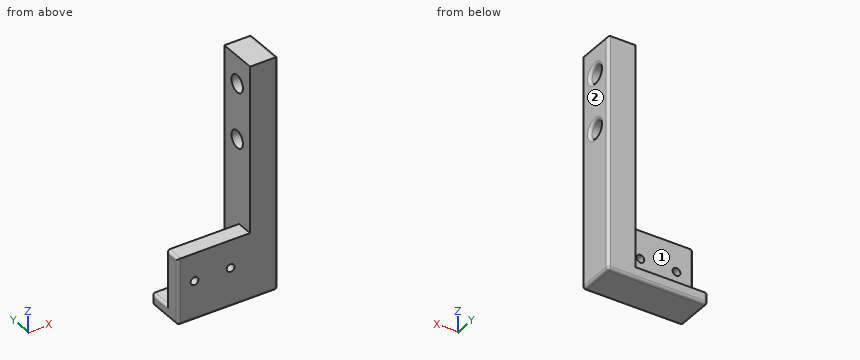
```python
from build123d import *

# Parameters (mm, degrees)
SKETCH_1_R          = 0.7
EXTRUDE_1_DEPTH     = 7
SKETCH_2_R          = 1.55
CUT_EXTRUDE_1_DEPTH = 32.591137998
SKETCH_3_W          = 13
SKETCH_3_H          = 10
CUT_EXTRUDE_2_DEPTH = 4
SKETCH_4_W          = 18
SKETCH_4_H          = 2
EXTRUDE_2_DEPTH     = 7
FILLET_1_R          = 0.5
FILLET_2_R          = 0.5


with BuildPart() as part:
    # 草图1 → 凸台-拉伸1 (new body)
    with BuildSketch(Plane(origin=(0, 0, 0), x_dir=(1, 0, 0), z_dir=(0, 1, 0))):
        Polygon((-2.5, 15), (-2.5, -15), (2.5, -15), (2.5, 15), (2.5, 25), (-15.5, 25), (-15.5, 15), align=None)
        with Locations(Location((-12.5, 20, 0), (0, 0, 270))):
            Circle(SKETCH_1_R, mode=Mode.SUBTRACT)
        with Locations(Location((-6, 20, 0), (0, 0, 270))):
            Circle(SKETCH_1_R, mode=Mode.SUBTRACT)
    extrude(amount=EXTRUDE_1_DEPTH)

    # 草图2 → 切除-拉伸1 (cut, through all)
    with BuildSketch(Plane(origin=(2.5, 0, 0), x_dir=(0, 0, -1), z_dir=(1, 0, 0))):
        with Locations((-10, 3.5)):
            Circle(SKETCH_2_R)
        with Locations((0, 3.5)):
            Circle(SKETCH_2_R)
    extrude(amount=-CUT_EXTRUDE_1_DEPTH, mode=Mode.SUBTRACT)

    # 草图3 → 切除-拉伸2 (cut)
    with BuildSketch(Plane(origin=(0, 7, 0), x_dir=(1, 0, 0), z_dir=(0, 1, 0))):
        with Locations((-9, 20)):
            Rectangle(SKETCH_3_W, SKETCH_3_H)
    extrude(amount=-CUT_EXTRUDE_2_DEPTH, mode=Mode.SUBTRACT)

    # 草图4 → 凸台-拉伸2 (add)
    with BuildSketch(Plane.XZ):
        with Locations((-6.5, -26)):
            Rectangle(SKETCH_4_W, SKETCH_4_H)
    extrude(amount=-EXTRUDE_2_DEPTH)

    # 圆角1
    fillet_1_edges = [part.edges().sort_by_distance(p)[0] for p in [
        (2.5, 3.5, 15),
        (2.5, 3.5, 11.55),
        (2.5, 3.5, 1.55),
        (2.5, 7, -6),
        (-15.5, 3.5, -27),
        (-6.5, 7, -27),
        (2.5, 3.5, -27),
        (-6.5, 0, -27),
        (2.5, 0, -6),
    ]]
    fillet(fillet_1_edges, radius=FILLET_1_R)

    # 圆角2
    # the kernel refuses this fillet: 0.5 mm, written as the material it takes off along each edge
    with BuildSketch(Plane(origin=(-15, 6.5, -26.5), x_dir=(-1, 0, 0), z_dir=(0, 1, 0))) as fillet_2_piece_1_section:
        Polygon((0, 0), (FILLET_2_R, 0), (FILLET_2_R, -FILLET_2_R), (0, -FILLET_2_R), align=None)
    fillet_2_piece_1 = extrude(amount=FILLET_2_R, mode=Mode.PRIVATE)
    fillet_2_piece_1 = fillet_2_piece_1 - Plane(origin=(-15, 6.5, -26.5), x_dir=(0.7071067811865475, 0, 0.7071067811865475), z_dir=(0, 1, 0)) * Sphere(FILLET_2_R, mode=Mode.PRIVATE)
    add(fillet_2_piece_1, mode=Mode.SUBTRACT)
    with BuildSketch(Plane(origin=(-15, 0.5, -26.5), x_dir=(-1, 0, 0), z_dir=(0, -1, 0))) as fillet_2_piece_2_section:
        Polygon((0, 0), (FILLET_2_R, 0), (FILLET_2_R, FILLET_2_R), (0, FILLET_2_R), align=None)
    fillet_2_piece_2 = extrude(amount=FILLET_2_R, mode=Mode.PRIVATE)
    fillet_2_piece_2 = fillet_2_piece_2 - Plane(origin=(-15, 0.5, -26.5), x_dir=(0.7071067811865475, 0, 0.7071067811865475), z_dir=(0, -1, 0)) * Sphere(FILLET_2_R, mode=Mode.PRIVATE)
    add(fillet_2_piece_2, mode=Mode.SUBTRACT)
    with BuildSketch(Plane(origin=(-15.5, -1.25, -15), x_dir=(1, 0, 0), z_dir=(0, 1, 0))) as fillet_2_piece_3:
        with BuildLine():
            CenterArc((FILLET_2_R, FILLET_2_R), FILLET_2_R, 180, 90)
            Line((0, FILLET_2_R), (0, 0))
            Line((0, 0), (FILLET_2_R, 0))
        make_face()
    extrude(amount=5.5, mode=Mode.SUBTRACT)
    with BuildSketch(Plane(origin=(-15.5, 3, -25), x_dir=(1, 0, 0), z_dir=(0, 0, 1))) as fillet_2_piece_4:
        with BuildLine():
            CenterArc((FILLET_2_R, -FILLET_2_R), FILLET_2_R, 90, 90)
            Line((0, -FILLET_2_R), (0, 0))
            Line((0, 0), (FILLET_2_R, 0))
        make_face()
    extrude(amount=11.25, mode=Mode.SUBTRACT)
    with BuildSketch(Plane(origin=(-15.5, 3, -25), x_dir=(1, 0, 0), z_dir=(0, 1, 0))) as fillet_2_piece_5:
        with BuildLine():
            CenterArc((FILLET_2_R, FILLET_2_R), FILLET_2_R, 180, 90)
            Line((0, FILLET_2_R), (0, 0))
            Line((0, 0), (FILLET_2_R, 0))
        make_face()
    extrude(amount=5.25, mode=Mode.SUBTRACT)
    with BuildSketch(Plane(origin=(-15.5, 7, -26.5), x_dir=(1, 0, 0), z_dir=(0, 0, 1))) as fillet_2_piece_6:
        with BuildLine():
            CenterArc((FILLET_2_R, -FILLET_2_R), FILLET_2_R, 90, 90)
            Line((0, -FILLET_2_R), (0, 0))
            Line((0, 0), (FILLET_2_R, 0))
        make_face()
    extrude(amount=2.75, mode=Mode.SUBTRACT)
    with BuildSketch(Plane(origin=(-15.5, 0, -13.75), x_dir=(1, 0, 0), z_dir=(0, 0, -1))) as fillet_2_piece_7:
        with BuildLine():
            CenterArc((FILLET_2_R, -FILLET_2_R), FILLET_2_R, 90, 90)
            Line((0, -FILLET_2_R), (0, 0))
            Line((0, 0), (FILLET_2_R, 0))
        make_face()
    extrude(amount=12.75, mode=Mode.SUBTRACT)
    with BuildSketch(Plane(origin=(-15.5, 3, -26.25), x_dir=(1, 0, 0), z_dir=(0, 0, 1))) as fillet_2_piece_8a_section:
        with BuildLine():
            CenterArc((FILLET_2_R, -FILLET_2_R), FILLET_2_R, 90, 90)
            Line((0, -FILLET_2_R), (0, 0))
            Line((0, 0), (FILLET_2_R, 0))
        make_face()
    fillet_2_piece_8a = extrude(amount=12.5, mode=Mode.PRIVATE)
    fillet_2_piece_8a = split(fillet_2_piece_8a, bisect_by=Plane(origin=(-15.386802443, 2.886802443, -25), z_dir=(0, 0, -1)), keep=Keep.TOP, mode=Mode.PRIVATE)
    with BuildSketch(Plane(origin=(-15.5, 1.75, -25), x_dir=(1, 0, 0), z_dir=(0, 1, 0))) as fillet_2_piece_8b_section:
        with BuildLine():
            CenterArc((FILLET_2_R, FILLET_2_R), FILLET_2_R, 180, 90)
            Line((0, FILLET_2_R), (0, 0))
            Line((0, 0), (FILLET_2_R, 0))
        make_face()
    fillet_2_piece_8b = extrude(amount=6.5, mode=Mode.PRIVATE)
    fillet_2_piece_8b = split(fillet_2_piece_8b, bisect_by=Plane(origin=(-15.386802443, 3, -25.113197557), z_dir=(0, -1, 0)), keep=Keep.TOP, mode=Mode.PRIVATE)
    fillet_2_piece_8 = fillet_2_piece_8a & fillet_2_piece_8b
    add(fillet_2_piece_8, mode=Mode.SUBTRACT)


solid = part.part
```
CAD build for the part. Positions are in the model's coordinates, mm. Face numbers are marked on the shaded views. Coordinates: 2 decimals unless noted, no trailing zeros. Write each loop counter-clockwise with the first axis right and the second up, starting at its lowest first coordinate (ties: lowest second). Pieces come first, ordered by that corner, then holes. Notation, with made-up numbers: (26.5, 19.25) -> (69.5, 19.25) arc R11 cw to (69.5, 37.25) -> close; hole circle Ø5 at (4, 61). An arc over 180 degrees is marked (long way). Return JSON: item names as keys, results as strings. Group by question number.
Q1. Flat gauge pins, fed straight in: pin 1 (1.8 mm diameter, centred on x = -6, z = -20, fed in from -Y); pin 2 (1.9 mm diameter, centred on y = 3.5, z = 10, fed in from +X); pin 3 (2 mm diameter, centred on x = -7, y = 5.5, fed in from +Z); pin 4 (0.9 mm diameter, centred on x = -7, y = 1.5, fed in from +Z). Where does each tip first touch, or does it go through?
Q2. Cut at A-A, the plane y = 3.5. Give the cut face in (x, z), then the cut area to 3 significant figures.
Q3. Pull direction X, two halves, no side cores. Call the marked faces 1 and 2: released by +X, released by -X, zero draft, split by the parting line, or undercut.
Q4. Cut at D-D, the plane z = -23. Give the cut face in (x, y), then the cut area to 3 significant figures.
Q5. Cut at B-B, the plane x = -12.5. Give the cut face in (y, z), then the cut area to 3 significant figures.
Q6. Drill centre lines: line 1 (X direction, y = 1.75, z = -20); line 2 (Y direction, x = -0.3, z = 0); line 3 (Z direction, x = -0.75, y = 4). Where is each one in solid material? Low to high.
Q7. Cut at C-C, the plane z = 0. Give the cut face in (x, y), then the cut area to 3 significant figures.
Returned:
{
 "1": {"pin 1": "stops at y = 0", "pin 2": "passes through", "pin 3": "stops at z = -25", "pin 4": "stops at z = -15"},
 "2": {"outline": "(-15.5, -26.5) arc R0.5 ccw to (-15, -27) -> (2, -27) arc R0.5 ccw to (2.5, -26.5) -> (2.5, -2.05) arc R0.5 ccw to (2, -1.55) -> (-2.5, -1.55) -> (-2.5, -25) -> (-15, -25) arc R0.5 ccw to (-15.5, -25.5) -> close; (-2.5, 1.55) -> (2, 1.55) arc R0.5 ccw to (2.5, 2.05) -> (2.5, 7.95) arc R0.5 ccw to (2, 8.45) -> (-2.5, 8.45) -> close; (-2.5, 11.55) -> (2, 11.55) arc R0.5 ccw to (2.5, 12.05) -> (2.5, 14.5) arc R0.5 ccw to (2, 15) -> (-2.5, 15) -> close", "area": "205 mm2"},
 "3": {"face 1": "zero draft", "face 2": "released by +X"},
 "4": {"outline": "(-15.5, 0.5) arc R0.5 ccw to (-15, 0) -> (2, 0) arc R0.5 ccw to (2.5, 0.5) -> (2.5, 6.5) arc R0.5 ccw to (2, 7) -> (-2.5, 7) -> (-2.5, 3) -> (-15, 3) arc R0.5 ccw to (-15.5, 2.5) -> close", "area": "73.8 mm2"},
 "5": {"outline": "(0, -26.5) arc R0.5 ccw to (0.5, -27) -> (6.5, -27) arc R0.5 ccw to (7, -26.5) -> (7, -25) -> (3, -25) -> (3, -20.7) -> (0, -20.7) -> close; (0, -19.3) -> (3, -19.3) -> (3, -15) -> (0, -15) -> close", "area": "39.7 mm2"},
 "6": {"line 1": "x = -15.5 to -13.2, -11.8 to -6.7, -5.3 to 2.5", "line 2": "y = 0 to 1.95, 5.05 to 7", "line 3": "z = -27 to -1.47, 1.47 to 8.53, 11.47 to 15"},
 "7": {"outline": "(-2.5, 0) -> (2, 0) arc R0.5 ccw to (2.5, 0.5) -> (2.5, 1.45) arc R0.5 ccw to (2, 1.95) -> (-2.5, 1.95) -> close; (-2.5, 5.05) -> (2, 5.05) arc R0.5 ccw to (2.5, 5.55) -> (2.5, 6.5) arc R0.5 ccw to (2, 7) -> (-2.5, 7) -> close", "area": "19.3 mm2"}
}
